Autodesk Inventor part; units mm, degrees
ref_plane "YZ Plane" through (0, 0, 0) normal (1, 0, 0) x (0, 1, 0)
ref_plane "XZ Plane" through (0, 0, 0) normal (0, 1, 0) x (-1, 0, 0)
ref_plane "XY Plane" through (0, 0, 0) normal (0, 0, 1) x (1, 0, 0)
sketch "Sketch1" plane through (0, 0, 0) normal (0, 0, 1) x (1, 0, 0)
  line L0 (-94.3346, 851.946) -> (-94.3346, 838.0325)
  line L1 (-94.3346, 838.0325) -> (-66.3346, 838.0325)
  line L2 (-66.3346, 838.0325) -> (-66.3346, 860.346)
  line L3 (-66.3346, 860.346) -> (-66.4468, 862.1155)
  line L4 (-66.4468, 862.1155) -> (-66.7819, 863.8566)
  line L5 (-66.7819, 863.8566) -> (-67.3343, 865.5414)
  line L6 (-67.3343, 865.5414) -> (-68.0952, 867.1429)
  line L7 (-68.0952, 867.1429) -> (-69.0524, 868.6354)
  line L8 (-69.0524, 868.6354) -> (-70.1906, 869.9949)
  line L9 (-70.1906, 869.9949) -> (-71.4915, 871.1996)
  line L10 (-71.4915, 871.1996) -> (-72.9342, 872.2303)
  line L11 (-72.9342, 872.2303) -> (-74.4956, 873.0703)
  line L12 (-74.4956, 873.0703) -> (-76.1507, 873.7063)
  line L13 (-76.1507, 873.7063) -> (-77.8729, 874.1279)
  line L14 (-77.8729, 874.1279) -> (-79.6346, 874.3285)
  line L15 (-79.6346, 874.3285) -> (-79.6346, 870.8227)
  line L16 (-79.6346, 870.8227) -> (-77.9981, 870.5828)
  line L17 (-77.9981, 870.5828) -> (-76.4195, 870.0889)
  line L18 (-76.4195, 870.0889) -> (-74.9382, 869.3532)
  line L19 (-74.9382, 869.3532) -> (-73.5907, 868.394)
  line L20 (-73.5907, 868.394) -> (-72.4106, 867.2352)
  line L21 (-72.4106, 867.2352) -> (-71.427, 865.9054)
  line L22 (-71.427, 865.9054) -> (-70.6646, 864.4376)
  line L23 (-70.6646, 864.4376) -> (-70.142, 862.8683)
  line L24 (-70.142, 862.8683) -> (-69.8724, 861.2365)
  line L25 (-69.8724, 861.2365) -> (-69.8623, 859.5825)
  line L26 (-69.8623, 859.5825) -> (-70.1122, 857.9475)
  line L27 (-70.1122, 857.9475) -> (-70.6156, 856.372)
  line L28 (-70.6156, 856.372) -> (-71.3603, 854.8951)
  line L29 (-71.3603, 854.8951) -> (-72.3276, 853.5535)
  line L30 (-72.3276, 853.5535) -> (-73.4936, 852.3804)
  line L31 (-73.4936, 852.3804) -> (-74.8293, 851.405)
  line L32 (-74.8293, 851.405) -> (-76.3017, 850.6514)
  line L33 (-76.3017, 850.6514) -> (-77.8741, 850.1384)
  line L34 (-77.8741, 850.1384) -> (-79.5076, 849.8787)
  line L35 (-79.5076, 849.8787) -> (-81.1615, 849.8787)
  line L36 (-81.1615, 849.8787) -> (-82.795, 850.1384)
  line L37 (-82.795, 850.1384) -> (-84.3674, 850.6514)
  line L38 (-84.3674, 850.6514) -> (-85.8398, 851.405)
  line L39 (-85.8398, 851.405) -> (-87.1755, 852.3804)
  line L40 (-87.1755, 852.3804) -> (-88.3415, 853.5535)
  line L41 (-88.3415, 853.5535) -> (-89.3088, 854.8951)
  line L42 (-89.3088, 854.8951) -> (-90.0535, 856.372)
  line L43 (-90.0535, 856.372) -> (-90.5569, 857.9475)
  line L44 (-90.5569, 857.9475) -> (-90.8068, 859.5825)
  line L45 (-90.8068, 859.5825) -> (-90.7967, 861.2365)
  line L46 (-90.7967, 861.2365) -> (-90.5271, 862.8683)
  line L47 (-90.5271, 862.8683) -> (-90.0046, 864.4376)
  line L48 (-90.0046, 864.4376) -> (-89.2421, 865.9054)
  line L49 (-89.2421, 865.9054) -> (-88.2586, 867.2352)
  line L50 (-88.2586, 867.2352) -> (-87.0784, 868.394)
  line L51 (-87.0784, 868.394) -> (-85.731, 869.3532)
  line L52 (-85.731, 869.3532) -> (-84.2496, 870.0889)
  line L53 (-84.2496, 870.0889) -> (-82.6711, 870.5828)
  line L54 (-82.6711, 870.5828) -> (-81.0346, 870.8227)
  line L55 (-81.0346, 870.8227) -> (-81.0346, 874.3285)
  line L56 (-81.0346, 874.3285) -> (-82.7962, 874.1279)
  line L57 (-82.7962, 874.1279) -> (-84.5184, 873.7063)
  line L58 (-84.5184, 873.7063) -> (-86.1735, 873.0703)
  line L59 (-86.1735, 873.0703) -> (-87.7349, 872.2303)
  line L60 (-87.7349, 872.2303) -> (-89.1776, 871.1996)
  line L61 (-89.1776, 871.1996) -> (-90.4785, 869.9949)
  line L62 (-90.4785, 869.9949) -> (-91.6167, 868.6354)
  line L63 (-91.6167, 868.6354) -> (-92.5739, 867.1429)
  line L64 (-92.5739, 867.1429) -> (-93.3349, 865.5414)
  line L65 (-93.3349, 865.5414) -> (-93.8873, 863.8566)
  line L66 (-93.8873, 863.8566) -> (-94.2223, 862.1155)
  line L67 (-94.2223, 862.1155) -> (-94.3346, 860.346)
  line L68 (-94.3346, 860.346) -> (-99.5495, 860.346)
  arc A0 (-99.5495, 860.346) -> (-101.5495, 858.346) centre (-99.5495, 858.346) ccw
  line L69 (-101.5495, 858.346) -> (-101.5495, 853.946)
  arc A1 (-101.5495, 853.946) -> (-99.5495, 851.946) centre (-99.5495, 853.946) ccw
  line L70 (-99.5495, 851.946) -> (-94.3346, 851.946)
  circle A2 centre (-98.0495, 856.146) radius 1.6
  circle A3 centre (-87.3346, 844.0325) radius 2.6
  circle A4 centre (-73.3346, 844.0325) radius 2.6
  point P0 (0, 0)
extrude "Extrusion1" add sketch "Sketch1" along normal blind 6
sketch "Sketch3" plane through (0, 0, 0) normal (0, 0, -1) x (-1, 0, 0)
  line L0 (69.8724, 861.2365) -> (69.8623, 859.5825)
  line L1 (69.8674, 860.4095) -> (90.8017, 860.4095)
  line L2 (90.8068, 859.5825) -> (90.7967, 861.2365)
  point P0 (0, 0)
  point P1 (80.3346, 860.4095)
hole "Hole1" at (-80.3346, 860.4095, 0) direction (0, 0, 1) diameter 21.2 depth 8 tip angle 118
properties part number "Left Bed Holder Upper"
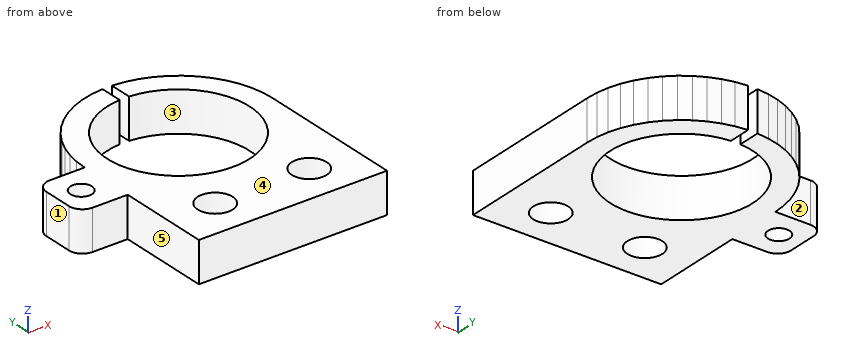
The listing builds one solid part. Answer for the finished solid, in the listing's coordinates (mm). Face numbers are marked on the shaded views. A direction names the side the tool comes from. Round coordinates to 2 decimals unless told otherwise and drop trailing zeros. Write each loop counter-clockwise with the first axis right and the second up, starting at its lowest first coordinate (ties: lowest second). Pieces come first, ordered by that corner, then holes. Notation, with made-up numbers: (11.25, 89.5) - (25.25, 89.5) arc R20 cw to (25.25, 99.5) - close; hole circle Ø1 at (3, 30.25). An arc over 180 degrees is marked (long way). Use a Markdown table: item, result. Add a question column.
1. Consider line 1 (X direction, y = 860.5, z = 2.1); line 2 (X direction, y = 856.5, z = 4.35); line 3 (X direction, y = 842.5, z = 1.3). Determine where each line is inside the solid, lowest interval first.
2. The part is cut by section D-D (x = -95). Write down the section's boundary in (y, z).
3. Flat-ended cylindrical pins translate along their axes: P1, Ø4, axis at x = -72.5, y = 843.5, coming from the +Z side; P2, Ø19, axis at x = -80.33, y = 860.41, coming from the -Z side (1 decimal); P3, Ø1, axis at x = -95.5, z = 3, coming from the +Y side; P4, Ø1.7, axis at y = 873, z = 2.5, coming from the -X side. Find the tip coordinate at first contact, or state that the pin passes through.
4. The part is cut by section A-A (y = 865). Write down the section's boundary in (x, z), and give its area (3 significant figures).
5. The part is cut by section B-B (x = -77). Write down the section's boundary in (y, z).
6. The part is cut by section C-C (y = 842.5). Write down the section's boundary in (x, z).
7. A tool of negligible diameter and unlimited length cuts with its end or side. For the marked faces 4 and 5, from which of +Z, -Z, +X, -X, +Y, -Y can it reach the whole face along a straight path? Write none if from no direction.
8. For a pull along X with two mould halves and no side action, classify the marked faces 1, 2 and 3 as +X half, -X half, draft (parallel to the pull), parting line (faces both ways), or undercut.
Reported:
| question | item | result |
|---|---|---|
| 1 | line 1 | -94.32 to -90.93, -69.73 to -66.34 |
| 1 | line 2 | -101.55 to -99.61, -96.49 to -90.19, -70.48 to -66.33 |
| 1 | line 3 | -94.33 to -89.43, -85.23 to -75.43, -71.23 to -66.33 |
| 2 | outline | (851.95, 0) - (860.35, 0) - (860.35, 6) - (851.95, 6) - close |
| 3 | P1 | z = 6 |
| 3 | P2 | through |
| 3 | P3 | y = 860.35 |
| 3 | P4 | x = -87.85 |
| 4 | outline | (-93.51, 0) - (-89.89, 0) - (-89.89, 6) - (-93.51, 6) - close; (-70.78, 0) - (-67.16, 0) - (-67.16, 6) - (-70.78, 6) - close |
| 4 | area | 43.5 mm^2 |
| 5 | outline | (838.03, 0) - (850.35, 0) - (850.35, 6) - (838.03, 6) - close; (870.47, 0) - (873.91, 0) - (873.91, 6) - (870.47, 6) - close |
| 6 | outline | (-94.33, 0) - (-89.43, 0) - (-89.43, 6) - (-94.33, 6) - close; (-85.23, 0) - (-75.43, 0) - (-75.43, 6) - (-85.23, 6) - close; (-71.23, 0) - (-66.33, 0) - (-66.33, 6) - (-71.23, 6) - close |
| 7 | face 4 | +Z, +X, -X, +Y, -Y |
| 7 | face 5 | +Z, -Z, -X, -Y |
| 8 | face 1 | -X half |
| 8 | face 2 | draft |
| 8 | face 3 | undercut |
